Source: three-view drawing plus pictorial views. Frame: mm from the lowest corner of the part. Give positions to 0.01 mm unless a question says otherwise; leave off trailing zeros. Loops run counter-clockwise (first coordinate to the right, second up) from the corner with the lowest first, then second, coordinate; pieces in that order, holes last. Notation, with made-up numbers: M -16.5,60.5 L 19.5,60.5 A14 cw 19.5,78.5 Z; hole C 69,73 d9. An arc over 180 degrees is marked long. One line per item, written item: value. Start each with the question number.
(1) Pin query (flat end, axial travel): P1, Ø7.5, axis at x = 25.4, z = 25.4, coming from the -Y side. Return the tip coordinate at first contact, or that it passes through.
(2) Section B-B on x = 29.5. Output: boundary loops of the cut face in (y, z) (1 decimal).
(3) Section D-D on x = 8. Output: boundary loops of the cut face in (y, z) (1 decimal).
(4) Ray query, line 1 along Z through (x, y) = (25, 1.3) (1 decimal); line 2 along Z through (x, y) = (29, 1.2) (1 decimal); line 3 along X through (y, z) = (0.3, 37.5). Return the intervals inside material, ascending. Write a range as from..to.
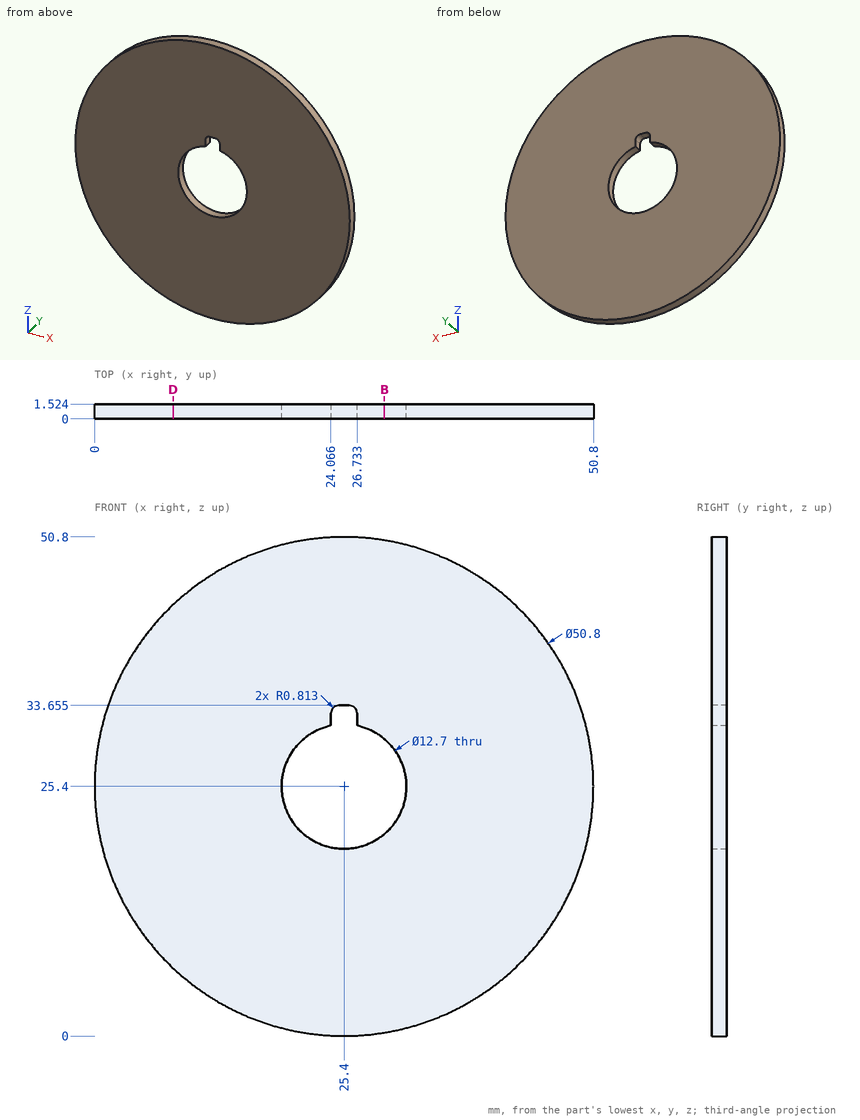
Output values:
1. P1: passes through
2. outline: M 0,0.3 L 1.5,0.3 L 1.5,20.6 L 0,20.6 Z; M 0,30.2 L 1.5,30.2 L 1.5,50.5 L 0,50.5 Z
3. outline: M 0,6.9 L 1.5,6.9 L 1.5,43.9 L 0,43.9 Z
4. line 1: z = 0..19.1, 33.7..50.8
4. line 2: z = 0.3..20.2, 30.6..50.5
4. line 3: x = 3.07..47.73
